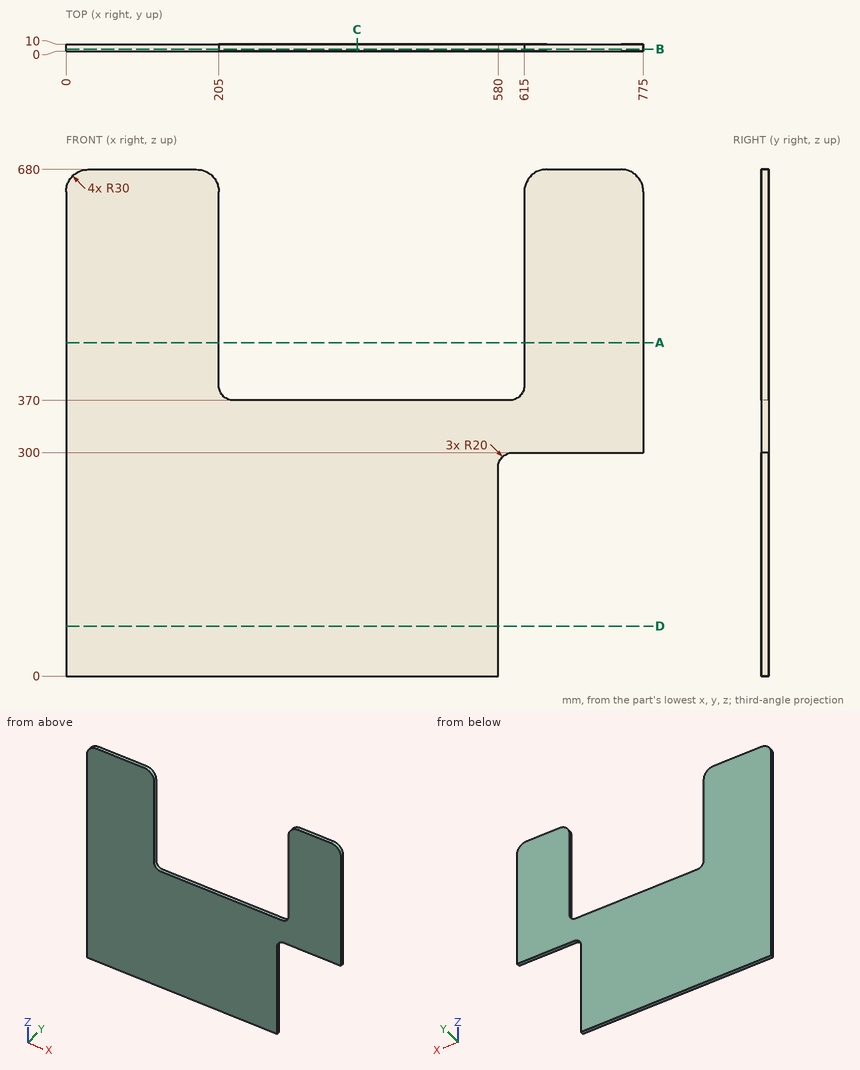
Verification items for this drawing (mm, ordinates from the low corner). Give positions to 0.01 mm unless a question says otherwise; leave off trailing zeros. Loops run counter-clockwise (first coordinate to the right, second up) from the corner with the lowest first, then second, coordinate; pieces in that order, holes last. Notation, with made-up numbers: M 80.25,52.25 L 98.25,52.25 A17 ccw 98.25,61.25 Z; hole C 80,-8.75 d7. An arc over 180 degrees is marked long. Write each question's results on one line, items separated by ' | '.
1) Section check B-B, the plane y = 3.25. Record the boundary of the cut face in (x, z).
Answers follow:
outline: M 0,0 L 580,0 L 580,280 A20 cw 600,300 L 775,300 L 775,650 A30 ccw 745,680 L 645,680 A30 ccw 615,650 L 615,390 A20 cw 595,370 L 225,370 A20 cw 205,390 L 205,650 A30 ccw 175,680 L 30,680 A30 ccw 0,650 Z
2) Gauge pin test, flat ends, axial feed: pin 1 (3 mm diameter, centred on y = 7, z = 170, fed in from +X); pin 2 (3 mm diameter, centred on x = 622.5, y = 8, fed in from -Z). Record the tip position at first contact, or that the pin passes through.
Answers follow:
pin 1: x = 580 | pin 2: z = 300
3) Thickness scan on line 1 (X direction, y = 2, z = 567); line 2 (X direction, y = 5, z = 652); line 3 (Z direction, x = 429.5, y = 4). Record the ranges inside material, lowest first.
Answers follow:
line 1: 0 to 205, 615 to 775 | line 2: 0.07 to 204.93, 615.07 to 774.93 | line 3: 0 to 370
4) Section check D-D, the plane z = 67. Record the boundary of the cut face in (x, y), plus the area to 3 significant figures.
Answers follow:
outline: M 0,0 L 580,0 L 580,10 L 0,10 Z | area: 5,800 mm2
5) Section check C-C, the plane x = 390.5. Record the boundary of the cut face in (y, z), plus the area to 3 significant figures.
Answers follow:
outline: M 0,0 L 10,0 L 10,370 L 0,370 Z | area: 3,700 mm2
6) Section check A-A, the plane z = 447.5. Record the boundary of the cut face in (x, y).
Answers follow:
outline: M 0,0 L 205,0 L 205,10 L 0,10 Z; M 615,0 L 775,0 L 775,10 L 615,10 Z
